For this review, take the finished solid that the model builds, in its own axes (mm). A direction names the side the tool comes from. Give positions to 0.01 mm unless a question says otherwise; leave off trailing zeros. Loops run counter-clockwise (first coordinate to the right, second up) from the corner with the lowest first, then second, coordinate; pieces in that order, holes last. Notation, with made-up numbers: (-15, 53) -> (38, 53) arc R8 cw to (38, 66) -> close; hole circle Ø11 at (24.5, 54). An arc over 180 degrees is marked (long way). Write each question's results on one line, items separated by ' | '. Start each with the question number.
```python
from build123d import *

# Parameters (mm, degrees)
EXTRUDE_2_DEPTH     = 3
SKETCH_2_R          = 5
EXTRUDE_3_DEPTH     = 25
EXTRUDE_START       = 58
SKETCH_3_R          = 5
EXTRUDE_4_DEPTH     = 58
SKETCH_4_R          = 15
EXTRUDE_5_DEPTH     = 3
SKETCH_5_R          = 1.5
CUT_EXTRUDE_1_DEPTH = 3
SKETCH_7_R          = 2
CUT_EXTRUDE_2_DEPTH = 90
SKETCH_9_W          = 0.2
SKETCH_9_H          = 1.1
CHAMFER_3_SIZE      = 0.5


with BuildPart() as part:
    # 草图1 → 凸台-拉伸2 (new body)
    with BuildSketch(Plane.XY):
        with BuildLine():
            ThreePointArc((-11.779760181, 14.271379579), (-12.466737886, 13.675360013), (-13.123601243, 13.046306581))
            ThreePointArc((-13.123601243, 13.046306581), (-12.803108373, 12.120767872), (-12.365117817, 11.24469604))
            ThreePointArc((-12.365117817, 11.24469604), (-12.142820781, 10.31561124), (-12.473009262, 9.419179367))
            ThreePointArc((-12.473009262, 9.419179367), (-13.244860059, 8.856275392), (-14.199312115, 8.815830257))
            ThreePointArc((-14.199312115, 8.815830257), (-15.161802274, 8.997352368), (-16.139716175, 9.052324938))
            ThreePointArc((-16.139716175, 9.052324938), (-16.564996707, 8.248388274), (-16.950263236, 7.424527004))
            ThreePointArc((-16.950263236, 7.424527004), (-16.317069389, 6.677263239), (-15.592181711, 6.018571022))
            ThreePointArc((-15.592181711, 6.018571022), (-15.049271757, 5.2325282), (-15.033334803, 4.277352535))
            ThreePointArc((-15.033334803, 4.277352535), (-15.549719866, 3.473635543), (-16.425109435, 3.091133726))
            ThreePointArc((-16.425109435, 3.091133726), (-17.388178129, 2.912706505), (-18.319914067, 2.610703653))
            ThreePointArc((-18.319914067, 2.610703653), (-18.426060932, 1.707425992), (-18.487698254, 0.800023914))
            ThreePointArc((-18.487698254, 0.800023914), (-17.627319769, 0.331957205), (-16.713435066, -0.020395362))
            ThreePointArc((-16.713435066, -0.020395362), (-15.923235192, -0.557236769), (-15.563325175, -1.442154458))
            ThreePointArc((-15.563325175, -1.442154458), (-15.754503841, -2.378138035), (-16.432604711, -3.051037542))
            ThreePointArc((-16.432604711, -3.051037542), (-17.266184176, -3.565316511), (-18.02590605, -4.183507626))
            ThreePointArc((-18.02590605, -4.183507626), (-17.798583527, -5.064133631), (-17.528267179, -5.932526839))
            ThreePointArc((-17.528267179, -5.932526839), (-16.556902937, -6.058181489), (-15.577446402, -6.056607239))
            ThreePointArc((-15.577446402, -6.056607239), (-14.64667748, -6.271743824), (-13.991402244, -6.966890501))
            ThreePointArc((-13.991402244, -6.966890501), (-13.831554774, -7.908730892), (-14.220785664, -8.781149285))
            ThreePointArc((-14.220785664, -8.781149285), (-14.812296375, -9.561823776), (-15.297399536, -10.412713019))
            ThreePointArc((-15.297399536, -10.412713019), (-14.767308791, -11.151753946), (-14.201546494, -11.863856968))
            ThreePointArc((-14.201546494, -11.863856968), (-13.250384619, -11.630129203), (-12.337637284, -11.274840748))
            ThreePointArc((-12.337637284, -11.274840748), (-11.392004814, -11.139217123), (-10.52986291, -11.550709376))
            ThreePointArc((-10.52986291, -11.550709376), (-10.040577591, -12.371205819), (-10.088370713, -13.325318158))
            ThreePointArc((-10.088370713, -13.325318158), (-10.357925871, -14.266953756), (-10.502894449, -15.23562382))
            ThreePointArc((-10.502894449, -15.23562382), (-9.741627174, -15.733268097), (-8.956828262, -16.192907475))
            ThreePointArc((-8.956828262, -16.192907475), (-8.154328435, -15.631363523), (-7.431561886, -14.970344538))
            ThreePointArc((-7.431561886, -14.970344538), (-6.598778773, -14.502277424), (-5.646207243, -14.574540946))
            ThreePointArc((-5.646207243, -14.574540946), (-4.893564768, -15.162880849), (-4.593465396, -16.069828976))
            ThreePointArc((-4.593465396, -16.069828976), (-4.504660083, -17.045252575), (-4.289915268, -18.000879201))
            ThreePointArc((-4.289915268, -18.000879201), (-3.400284827, -18.18991721), (-2.502440741, -18.335016099))
            ThreePointArc((-2.502440741, -18.335016099), (-1.956985011, -17.521495584), (-1.521812876, -16.644020345))
            ThreePointArc((-1.521812876, -16.644020345), (-0.914351093, -15.9067248), (0, -15.63))
            ThreePointArc((0, -15.63), (0.914351093, -15.9067248), (1.521812876, -16.644020345))
            ThreePointArc((1.521812876, -16.644020345), (1.956985011, -17.521495584), (2.502440741, -18.335016099))
            ThreePointArc((2.502440741, -18.335016099), (3.400284827, -18.18991721), (4.289915268, -18.000879201))
            ThreePointArc((4.289915268, -18.000879201), (4.504660083, -17.045252575), (4.593465396, -16.069828976))
            ThreePointArc((4.593465396, -16.069828976), (4.893564768, -15.162880849), (5.646207243, -14.574540946))
            ThreePointArc((5.646207243, -14.574540946), (6.598778773, -14.502277424), (7.431561886, -14.970344538))
            ThreePointArc((7.431561886, -14.970344538), (8.154328435, -15.631363523), (8.956828262, -16.192907475))
            ThreePointArc((8.956828262, -16.192907475), (9.741627174, -15.733268097), (10.502894449, -15.23562382))
            ThreePointArc((10.502894449, -15.23562382), (10.357925871, -14.266953756), (10.088370713, -13.325318158))
            ThreePointArc((10.088370713, -13.325318158), (10.040577591, -12.371205819), (10.52986291, -11.550709376))
            ThreePointArc((10.52986291, -11.550709376), (11.392004814, -11.139217123), (12.337637284, -11.274840748))
            ThreePointArc((12.337637284, -11.274840748), (13.250384619, -11.630129203), (14.201546494, -11.863856968))
            ThreePointArc((14.201546494, -11.863856968), (14.767308791, -11.151753946), (15.297399536, -10.412713019))
            ThreePointArc((15.297399536, -10.412713019), (14.812296375, -9.561823776), (14.220785664, -8.781149285))
            ThreePointArc((14.220785664, -8.781149285), (13.831554774, -7.908730892), (13.991402244, -6.966890501))
            ThreePointArc((13.991402244, -6.966890501), (14.64667748, -6.271743824), (15.577446402, -6.056607239))
            ThreePointArc((15.577446402, -6.056607239), (16.556902937, -6.058181489), (17.528267179, -5.932526839))
            ThreePointArc((17.528267179, -5.932526839), (17.798583527, -5.064133631), (18.02590605, -4.183507626))
            ThreePointArc((18.02590605, -4.183507626), (17.266184176, -3.565316511), (16.432604711, -3.051037542))
            ThreePointArc((16.432604711, -3.051037542), (15.754503841, -2.378138035), (15.563325175, -1.442154458))
            ThreePointArc((15.563325175, -1.442154458), (15.923235192, -0.557236769), (16.713435066, -0.020395362))
            ThreePointArc((16.713435066, -0.020395362), (17.627319769, 0.331957205), (18.487698254, 0.800023914))
            ThreePointArc((18.487698254, 0.800023914), (18.426060932, 1.707425992), (18.319914067, 2.610703653))
            ThreePointArc((18.319914067, 2.610703653), (17.388178129, 2.912706505), (16.425109435, 3.091133726))
            ThreePointArc((16.425109435, 3.091133726), (15.549719866, 3.473635543), (15.033334803, 4.277352535))
            ThreePointArc((15.033334803, 4.277352535), (15.049271757, 5.2325282), (15.592181711, 6.018571022))
            ThreePointArc((15.592181711, 6.018571022), (16.317069389, 6.677263239), (16.950263236, 7.424527004))
            ThreePointArc((16.950263236, 7.424527004), (16.564996707, 8.248388274), (16.139716175, 9.052324938))
            ThreePointArc((16.139716175, 9.052324938), (15.161802274, 8.997352368), (14.199312115, 8.815830257))
            ThreePointArc((14.199312115, 8.815830257), (13.244860059, 8.856275392), (12.473009262, 9.419179367))
            ThreePointArc((12.473009262, 9.419179367), (12.142820781, 10.31561124), (12.365117817, 11.24469604))
            ThreePointArc((12.365117817, 11.24469604), (12.803108373, 12.120767872), (13.123601243, 13.046306581))
            ThreePointArc((13.123601243, 13.046306581), (12.466737886, 13.675360013), (11.779760181, 14.271379579))
            ThreePointArc((11.779760181, 14.271379579), (10.887741008, 13.866855937), (10.055819013, 13.349900061))
            ThreePointArc((10.055819013, 13.349900061), (9.151208508, 13.042826175), (8.228134706, 13.288893831))
            ThreePointArc((8.228134706, 13.288893831), (7.596414573, 14.005513822), (7.468076245, 14.952162548))
            ThreePointArc((7.468076245, 14.952162548), (7.560016626, 15.927295641), (7.524524182, 16.906110163))
            ThreePointArc((7.524524182, 16.906110163), (6.684777033, 17.255398605), (5.8288823, 17.563005328))
            ThreePointArc((5.8288823, 17.563005328), (5.143229987, 16.863563773), (4.554231832, 16.080991887))
            ThreePointArc((4.554231832, 16.080991887), (3.821635541, 15.46787101), (2.872004963, 15.363869548))
            ThreePointArc((2.872004963, 15.363869548), (2.024070484, 15.803894155), (1.562429593, 16.640256651))
            ThreePointArc((1.562429593, 16.640256651), (1.295902743, 17.582753877), (0.909218435, 18.482649887))
            ThreePointArc((0.909218435, 18.482649887), (0, 18.505), (-0.909218435, 18.482649887))
            ThreePointArc((-0.909218435, 18.482649887), (-1.295902743, 17.582753877), (-1.562429593, 16.640256651))
            ThreePointArc((-1.562429593, 16.640256651), (-2.024070484, 15.803894155), (-2.872004963, 15.363869548))
            ThreePointArc((-2.872004963, 15.363869548), (-3.821635541, 15.46787101), (-4.554231832, 16.080991887))
            ThreePointArc((-4.554231832, 16.080991887), (-5.143229987, 16.863563773), (-5.8288823, 17.563005328))
            ThreePointArc((-5.8288823, 17.563005328), (-6.684777033, 17.255398605), (-7.524524182, 16.906110163))
            ThreePointArc((-7.524524182, 16.906110163), (-7.560016626, 15.927295641), (-7.468076245, 14.952162548))
            ThreePointArc((-7.468076245, 14.952162548), (-7.596414573, 14.005513822), (-8.228134706, 13.288893831))
            ThreePointArc((-8.228134706, 13.288893831), (-9.151208508, 13.042826175), (-10.055819013, 13.349900061))
            ThreePointArc((-10.055819013, 13.349900061), (-10.887741008, 13.866855937), (-11.779760181, 14.271379579))
        make_face()
    extrude(amount=EXTRUDE_2_DEPTH)

    # 草图2 → 凸台-拉伸3 (add)
    with BuildSketch(Plane(origin=(0, 0, 0), x_dir=(-1, 0, 0), z_dir=(0, 0, -1))):
        with Locations(Location((0, 0, 0), (0, 0, 180))):
            Circle(SKETCH_2_R)
    extrude(amount=EXTRUDE_3_DEPTH)

    # 草图3 → 凸台-拉伸4 (add)
    with BuildSketch(Plane.XY.offset(3).offset(EXTRUDE_START)):
        Circle(SKETCH_3_R)
    extrude(amount=-EXTRUDE_4_DEPTH)

    # 草图4 → 凸台-拉伸5 (add)
    with BuildSketch(Plane(origin=(0, 0, 21.5), x_dir=(-1, 0, 0), z_dir=(0, 0, -1))):
        Circle(SKETCH_4_R)
    extrude(amount=-EXTRUDE_5_DEPTH)

    # 草图5 → 切除-拉伸1 (cut)
    with BuildSketch(Plane.XY.offset(24.5)):
        with Locations((0, 10)):
            Circle(SKETCH_5_R)
        with Locations((10, 0)):
            Circle(SKETCH_5_R)
        with Locations((0, -10)):
            Circle(SKETCH_5_R)
        with Locations((-10, 0)):
            Circle(SKETCH_5_R)
    extrude(amount=-CUT_EXTRUDE_1_DEPTH, mode=Mode.SUBTRACT)

    # 草图7 → 切除-拉伸2 (cut)
    with BuildSketch(Plane(origin=(0, 0, -25), x_dir=(-1, 0, 0), z_dir=(0, 0, -1))):
        Circle(SKETCH_7_R)
    extrude(amount=-CUT_EXTRUDE_2_DEPTH, mode=Mode.SUBTRACT)

    # 草图9 → 切除-旋转2 (revolve, cut)
    with BuildSketch(Plane(origin=(0, 0, 0), x_dir=(1, 0, 0), z_dir=(0, 1, 0)), mode=Mode.PRIVATE) as cut_revolve_2_sk:
        with Locations((4.9, 22.55)):
            Rectangle(SKETCH_9_W, SKETCH_9_H)
        with Locations((4.9, -58.55)):
            Rectangle(SKETCH_9_W, SKETCH_9_H)
    revolve(cut_revolve_2_sk.sketch.rotate(Axis((0, 0, -25), (0, 0, 1)), 180), axis=Axis((0, 0, -25), (0, 0, 1)), mode=Mode.SUBTRACT)

    # 倒角3
    chamfer_3_edges = [part.edges().sort_by_distance(p)[0] for p in [
        (-5, 0, -25),
        (-5, 0, 61),
    ]]
    chamfer(chamfer_3_edges, length=CHAMFER_3_SIZE)


solid = part.part
```
1. Machinability: for faces 4 (the cylindrical face through (-11.5, 0.07, 23.02)), 5 (the cylindrical face through (-1.08, -4.88, 12.38)), 6 (the cylindrical face through (17.615, 0.326, 1.479)), 7 (the cylindrical face through (6.7, 17.25, 1.48)), 8 (the cylindrical face through (-8.165, -15.64, 1.479)), which of the approach directions +Z, -Z, +X, -X, +Y, -Y give a long, thin tool a straight path to every point of the face, cutting with its end or side? Answer none if there is none.
2. Wall thickness on L1, parallel to Y at x = 0, z = 23; L2, parallel to Z at x = -12, y = 6; L3, parallel to X at y = 14, z = 2: over which ranges is each line inside the solid? List them lowest first.
3. For pin 1 Ø11 at (x, y) = (-1, -1.5) entering from +Z; pin 2 Ø2.5 at (x, y) = (-10, 0) entering from -Z; pin 3 Ø3 at (y, z) = (-2, 3.5) entering from +X; pin 4 Ø12 at (y, z) = (15, 22.5) entering from +X, all flat-tipped, find the tip position at first contact; note any pin that passes through.
4. We need section A-A (z = 23). Write out the cut boundary in (x, y).
5. Draft analysis for pull direction X (two halves, no side actions). For faces 1 (the cylindrical face through (10.36, -14.28, 1.48)), 2 (the flat face through (4, 4, 0)), 3 (the cylindrical face through (1.3, 17.57, 1.48)), state which applies: released by +X, released by -X, zero draft, split by the parting line, or undercut.
6. We need section B-B (z = 44). Write out the cut boundary in (x, y).
Response:
1) face 4: +Z | face 5: none | face 6: +Z, -Z, +X | face 7: +Z, -Z, +X, +Y | face 8: +Z, -Z, -Y
2) L1: y = -15 to -11.5, -8.5 to -2, 2 to 8.5, 11.5 to 15 | L2: z = 0 to 3, 21.5 to 24.5 | L3: x = -12.1 to -11.15, -7.6 to 7.6, 11.15 to 12.1
3) pin 1: stops at z = 61 | pin 2: stops at z = 0 | pin 3: stops at x = 17.05 | pin 4: stops at x = 12
4) outline: circle Ø30 at (0, 0); hole circle Ø3 at (-10, 0); hole circle Ø4 at (0, 0); hole circle Ø3 at (0, -10); hole circle Ø3 at (0, 10); hole circle Ø3 at (10, 0)
5) face 1: released by +X | face 2: zero draft | face 3: undercut
6) outline: circle Ø10 at (0, 0); hole circle Ø4 at (0, 0)
